Build history of the part. All positions in model axes, mm. A direction names the side the tool comes from. Round coordinates to 2 decimals unless told otherwise and drop trailing zeros. Write each loop counter-clockwise with the first axis right and the second up, starting at its lowest first coordinate (ties: lowest second). Pieces come first, ordered by that corner, then holes. Notation, with made-up numbers: (40, -9) - (64, -9) arc R14 ccw to (64, 8) - close; hole circle Ø5 at (75, 60). An arc over 180 degrees is marked (long way). Answer as a JSON object with one key per item and string values. Group by question number.
Item 1: Probe line 1 (Y direction, x = 44.07, z = 0.7); line 2 (Y direction, x = -48.26, z = 0.45); line 3 (Z direction, x = 19, y = -14.5). List the from-to ranges inside material, lowest first. Write a range as from..to.
Item 2: Two-plate mould, pull along Y, no slides. Class faces 1 (the flat face through (6, -57.25, 18)), 2 (the cylindrical face through (-46.568, 14.71, 0.986)), 3 (the flat face through (-2.65, -38, 10)): +Y half, -Y half, draft (parallel to the pull), parting line (faces both ways), or undercut.
Item 3: Slice it at D-D, the plane x = 7. List the corners of the cut face in (y, z).
Item 4: Flat gauge pins, fed straight in: pin 1 (1.6 mm diameter, centred on y = -56.5, z = 17, fed in from -X); pin 2 (4 mm diameter, centred on x = 28.5, y = -0.5, fed in from +Z); pin 3 (4 mm diameter, centred on x = 48.26, y = -36.2, fed in from -Z); pin 4 (10 mm diameter, centred on y = -24, z = 14.5, fed in from -X). Where does each tip first touch, or does it go through?
Item 5: Which spindle directions (+Z, -Z, +X, -X, +Y, -Y) get a long thin tool onto all of the face, cutting with end or side? Do faces 4 (the cylindrical face through (-46.568, -46.25, 0.986)), 5 (the flat face through (15.35, -38, 10)), 6 (the flat face through (6, -19.75, 10)). Say none if no direction does.
Item 6: Slice it at B-B, the plane x = -48.26. List the corners of the cut face in (y, z), then the cut area to 3 significant figures.
Item 7: Slice it at A-A, the plane y = 14.6. List the corners of the cut face in (x, z), then the cut area to 3 significant figures.
Item 8: Slice it at C-C, the plane x = 44.07. List the corners of the cut face in (y, z).
from build123d import *

# Parameters (mm, degrees)
F0_W     = 104.14
F0_H     = 110.5
F0_R     = 2.5
F0_R_2   = 1.5
F1_DEPTH = 2
F3_W     = 18
F3_H     = 35.5
F4_DEPTH = 17
F6_W     = 8
F6_H     = 3
F7_DEPTH = 2


with BuildPart() as f1:
    # F0 (on Top) → F1 (new body)
    with BuildSketch(Plane.XY):
        Rectangle(F0_W, F0_H)
        with Locations((-44.07, -46.36)):
            Circle(F0_R, mode=Mode.SUBTRACT)
        with Locations((-48.26, -36.2)):
            Circle(F0_R_2, mode=Mode.SUBTRACT)
        with Locations((-44.07, -26.04)):
            Circle(F0_R, mode=Mode.SUBTRACT)
        with Locations((-44.07, -5.72)):
            Circle(F0_R, mode=Mode.SUBTRACT)
        with Locations((44.07, -46.36)):
            Circle(F0_R, mode=Mode.SUBTRACT)
        with Locations((48.26, -36.2)):
            Circle(F0_R_2, mode=Mode.SUBTRACT)
        with Locations((44.07, -26.04)):
            Circle(F0_R, mode=Mode.SUBTRACT)
        with Locations((44.07, -5.72)):
            Circle(F0_R, mode=Mode.SUBTRACT)
        with Locations((-44.07, 14.6)):
            Circle(F0_R, mode=Mode.SUBTRACT)
        with Locations((-48.26, 25.4)):
            Circle(F0_R_2, mode=Mode.SUBTRACT)
        with Locations((44.07, 14.6)):
            Circle(F0_R, mode=Mode.SUBTRACT)
        with Locations((48.26, 25.4)):
            Circle(F0_R_2, mode=Mode.SUBTRACT)
    extrude(amount=F1_DEPTH)

    # F3 (on offset) → F4 (join)
    with BuildSketch(Plane.XY.offset(2)):
        with Locations((6.35, -37.5)):
            Rectangle(F3_W, F3_H)
    extrude(amount=F4_DEPTH)

    # F6 (on offset) → F7 (join)
    with BuildSketch(Plane.XZ.offset(55.25)):
        with Locations((6.35, 17.5)):
            Rectangle(F6_W, F6_H)
    extrude(amount=F7_DEPTH)


solid = f1.part
Geometry says:
{
 "1": {"line 1": "y = -55.25..-48.86, -43.86..-28.54, -23.54..-8.22, -3.22..12.1, 17.1..55.25", "line 2": "y = -55.25..-37.7, -34.7..23.9, 26.9..55.25", "line 3": "z = 0..2"},
 "2": {"face 1": "-Y half", "face 2": "undercut", "face 3": "draft"},
 "3": {"outline": "(-57.25, 16) - (-55.25, 16) - (-55.25, 0) - (55.25, 0) - (55.25, 2) - (-19.75, 2) - (-19.75, 19) - (-57.25, 19) - close"},
 "4": {"pin 1": "stops at x = 2.35", "pin 2": "stops at z = 2", "pin 3": "stops at z = 0", "pin 4": "stops at x = -2.65"},
 "5": {"face 4": "+Z, -Z", "face 5": "+Z, +X, +Y, -Y", "face 6": "+Z, +X, -X, +Y"},
 "6": {"outline": "(-55.25, 0) - (-37.7, 0) - (-37.7, 2) - (-55.25, 2) - close; (-34.7, 0) - (23.9, 0) - (23.9, 2) - (-34.7, 2) - close; (26.9, 0) - (55.25, 0) - (55.25, 2) - (26.9, 2) - close", "area": "209 mm^2"},
 "7": {"outline": "(-52.07, 0) - (-46.57, 0) - (-46.57, 2) - (-52.07, 2) - close; (-41.57, 0) - (41.57, 0) - (41.57, 2) - (-41.57, 2) - close; (46.57, 0) - (52.07, 0) - (52.07, 2) - (46.57, 2) - close", "area": "188 mm^2"},
 "8": {"outline": "(-55.25, 0) - (-48.86, 0) - (-48.86, 2) - (-55.25, 2) - close; (-43.86, 0) - (-28.54, 0) - (-28.54, 2) - (-43.86, 2) - close; (-23.54, 0) - (-8.22, 0) - (-8.22, 2) - (-23.54, 2) - close; (-3.22, 0) - (12.1, 0) - (12.1, 2) - (-3.22, 2) - close; (17.1, 0) - (55.25, 0) - (55.25, 2) - (17.1, 2) - close"}
}
